from build123d import *

# Parameters (mm, degrees)
CROQUIS1_W              = 52.23
CROQUIS1_H              = 10
CROQUIS1_W_2            = 10
SALIENTE_EXTRUIR1_DEPTH = 3


with BuildPart() as part:
    # Croquis1 → Saliente-Extruir1 (new body)
    with BuildSketch(Plane(origin=(0, 0, 0), x_dir=(1, 0, 0), z_dir=(0, 1, 0))):
        Polygon((17, 33.65), (17, 30.65), (8.5, 30.65), (8.5, 33.65), (0, 33.65), (0, 31.85), (3, 31.85), (3, 26.85), (0, 26.85), (0, 6.8), (3, 6.8), (3, 1.8), (0, 1.8), (0, 0), (8.5, 0), (8.5, 3), (17, 3), (17, 0), (30.865, 0), (30.865, 3), (39.365, 3), (39.365, 0), (53.23, 0), (53.23, 3), (61.73, 3), (61.73, 0), (70.23, 0), (70.23, 1.8), (67.23, 1.8), (67.23, 6.8), (70.23, 6.8), (70.23, 26.85), (67.23, 26.85), (67.23, 31.85), (70.23, 31.85), (70.23, 33.65), (61.73, 33.65), (61.73, 30.65), (53.23, 30.65), (53.23, 33.65), align=None)
        with Locations((35.115, 9)):
            Rectangle(CROQUIS1_W, CROQUIS1_H, mode=Mode.SUBTRACT)
        with Locations((35.115, 24.65)):
            Rectangle(CROQUIS1_W_2, CROQUIS1_H, mode=Mode.SUBTRACT)
    extrude(amount=SALIENTE_EXTRUIR1_DEPTH)


solid = part.part
For this review, take the finished solid that the model builds, in its own axes (mm). A direction names the side the tool comes from. Round coordinates to 2 decimals unless told otherwise and drop trailing zeros. Loops run counter-clockwise (first coordinate to the right, second up) from the corner with the lowest first, then second, coordinate; pieces in that order, holes last. Notation, with made-up numbers: (-2, 79.5) - (55, 79.5) arc R19 cw to (55, 113.5) - close; hole circle Ø2 at (85, 6). An arc over 180 degrees is marked (long way). One line per question, with ' | ' between items.
Q1. Take a section at C-C (x = 35). Give the boundary of the cut face in (y, z).
Taken from the geometry:
outline: (0, -33.65) - (3, -33.65) - (3, -29.65) - (0, -29.65) - close; (0, -19.65) - (3, -19.65) - (3, -14) - (0, -14) - close; (0, -4) - (3, -4) - (3, -3) - (0, -3) - close
Q2. Tool access review of faces 1 (the flat face through (67.23, 1, -29)), 2 (the flat face through (40.115, 1, -25)), 3 (the flat face through (8.5, 1, -1)): name each direction out of +Z, -Z, +X, -X, +Y, -Y from which nothing blocks a thin tool from reaching the whole face with its end or side.
Taken from the geometry:
face 1: +X, +Y, -Y | face 2: +Y, -Y | face 3: +Z, +Y, -Y
Q3. Take a section at B-B (x = 22). Give the boundary of the cut face in (y, z).
Taken from the geometry:
outline: (0, -33.65) - (3, -33.65) - (3, -14) - (0, -14) - close; (0, -4) - (3, -4) - (3, 0) - (0, 0) - close
Q4. Take a section at D-D (y = 2.25). State how many separate pieces and enclosed holes the cut face has, and give its area (3 significant figures).
Taken from the geometry:
separate pieces: 1 | enclosed holes: 2 | area: 1,550 mm²
Q5. For pin 1 (0.9 mm diameter, centred on x = 1, y = 1, fed in from +Z), flat-tipped, find the tip position at first contact; note if it passes through.
Taken from the geometry:
pin 1: stops at z = 0
Q6. The part is to be moulded in two halves that separate along X. For faces 4 (the flat face through (69, 1, -6.8)), 5 (the flat face through (35, 1, -3)), 6 (the flat face through (3, 1, -29)), say which applies: released by +X, released by -X, zero draft, split by the parting line, or undercut.
Taken from the geometry:
face 4: zero draft | face 5: undercut | face 6: released by -X
Q7. For line 1 along Z through (x, y) = (32, 2.65); line 2 along X through (y, z) = (2.55, -4.5); line 3 along Z through (x, y) = (49.5, 1.7), list the stretches that pass through material, from the lowest coordinate up. Write a range as [from, to].
Taken from the geometry:
line 1: z = [-33.65, -29.65], [-19.65, -14], [-4, -3] | line 2: x = [3, 9], [61.23, 67.23] | line 3: z = [-33.65, -14], [-4, 0]
Q8. Take a section at A-A (z = -25). Give the boundary of the cut face in (x, y) (3 decimals), and give its area (3 significant figures).
Taken from the geometry:
outline: (0, 0) - (30.115, 0) - (30.115, 3) - (0, 3) - close; (40.115, 0) - (70.23, 0) - (70.23, 3) - (40.115, 3) - close | area: 181 mm²
